```python
from build123d import *

# Parameters (mm, degrees)
SKETCH1_W               = 100
SKETCH1_H               = 100
BOSS_EXTRUDE1_DEPTH     = 50
SHELL1_T                = -10
CUT_EXTRUDE1_DEPTH      = 151
CUT_EXTRUDE1_DEPTH_BACK = 10
SKETCH2_W               = 50
SKETCH2_H               = 15
SKETCH3_W               = 25
SKETCH3_H               = 65
CUT_EXTRUDE2_DEPTH      = 10
SKETCH4_W               = 12.5
SKETCH4_H               = 32.5
CUT_EXTRUDE3_DEPTH      = 10
CUT_EXTRUDE4_START      = -40
SKETCH5_W               = 90
SKETCH5_H               = 90
CUT_EXTRUDE4_DEPTH      = 40
SKETCH6_W               = 6
SKETCH6_H               = 3
BOSS_EXTRUDE2_DEPTH     = 3


with BuildPart() as part:
    # Sketch1 → Boss-Extrude1 (new body)
    with BuildSketch(Plane.XY):
        with Locations((50, 50)):
            Rectangle(SKETCH1_W, SKETCH1_H)
    extrude(amount=BOSS_EXTRUDE1_DEPTH)

    # Shell1
    shell1_openings = [part.faces().sort_by_distance(p)[0] for p in [
        (50, 50, 50),
    ]]
    offset(amount=SHELL1_T, openings=shell1_openings, kind=Kind.INTERSECTION)

    # Sketch2 → Cut-Extrude1 (cut, two sides: drawn at the far end of the back side and taken through both)
    with BuildSketch(Plane.XZ.offset(-CUT_EXTRUDE1_DEPTH_BACK)):
        with Locations((50, 17.5)):
            Rectangle(SKETCH2_W, SKETCH2_H)
    extrude(amount=CUT_EXTRUDE1_DEPTH + CUT_EXTRUDE1_DEPTH_BACK, mode=Mode.SUBTRACT)

    # Sketch3 → Cut-Extrude2 (cut)
    with BuildSketch(Plane.ZY.offset(-100)):
        with Locations((22.5, 59.5)):
            Rectangle(SKETCH3_W, SKETCH3_H)
    extrude(amount=CUT_EXTRUDE2_DEPTH, mode=Mode.SUBTRACT)

    # Sketch4 → Cut-Extrude3 (cut)
    with BuildSketch(Plane(origin=(0, 0, 0), x_dir=(0, 0, -1), z_dir=(1, 0, 0))):
        with Locations((-16.25, 43.25)):
            Rectangle(SKETCH4_W, SKETCH4_H)
    extrude(amount=CUT_EXTRUDE3_DEPTH, mode=Mode.SUBTRACT)

    # Sketch5 → Cut-Extrude4 (cut)
    with BuildSketch(Plane.XY.offset(50).offset(CUT_EXTRUDE4_START)):
        with Locations((50, 50)):
            Rectangle(SKETCH5_W, SKETCH5_H)
    extrude(amount=CUT_EXTRUDE4_DEPTH, mode=Mode.SUBTRACT)

    # Sketch6 → Boss-Extrude2 (add)
    with BuildSketch(Plane.XY.offset(10)):
        with Locations((8, 31.5)):
            Rectangle(SKETCH6_W, SKETCH6_H)
        with Locations((92, 31.5)):
            Rectangle(SKETCH6_W, SKETCH6_H)
    extrude(amount=BOSS_EXTRUDE2_DEPTH)


solid = part.part
```
Build history of the part. All positions in model axes, mm. A direction names the side the tool comes from. Give positions to 0.01 mm unless a question says otherwise; leave off trailing zeros. Loops run counter-clockwise (first coordinate to the right, second up) from the corner with the lowest first, then second, coordinate; pieces in that order, holes last.
Item 1: Which spindle directions (+Z, -Z, +X, -X, +Y, -Y) get a long thin tool onto all of the face, cutting with end or side? Do faces 5 (the face through (2, 27, 16)), 6 (the face through (5, 49, 34)), 7 (the face through (92, 30, 11)), 8 (the face through (5, 31, 11)), 9 (the face through (75, 3, 17)). Say none if no direction does.
Answers follow:
face 5: +X, -X
face 6: +Z
face 7: +Z, +X, -X
face 8: -X
face 9: -Y
Item 2: Flat gauge pins, fed straight in: pin 1 (3.5 mm diameter, centred on y = 31, z = 12, fed in from -X); pin 2 (3 mm diameter, centred on y = 63.5, z = 17.5, fed in from +X); pin 3 (1.5 mm diameter, centred on x = 65.5, z = 17, fed in from -Y). Where does each tip first touch, or does it go through?
Answers follow:
pin 1: stops at x = 5
pin 2: stops at x = 5
pin 3: stops at y = 95
Item 3: Drill centre lines: line 1 (Y direction, x = 74, z = 46.5); line 2 (X direction, y = 84, z = 14). Where is each one in solid material? Low to high.
Answers follow:
line 1: y = 0 to 5, 95 to 100
line 2: x = 0 to 5
Item 4: Slice it at D-D, the plane z = 43.5. List the corners of the cut face in (x, y).
Answers follow:
outline: (0, 0) - (100, 0) - (100, 100) - (0, 100) - close; hole (5, 5) - (95, 5) - (95, 95) - (5, 95) - close
Item 5: Slice it at C-C, the plane y = 65. List the corners of the cut face in (x, z), and give its area (4 significant figures).
Answers follow:
outline: (0, 0) - (100, 0) - (100, 10) - (5, 10) - (5, 50) - (0, 50) - close; (95, 35) - (100, 35) - (100, 50) - (95, 50) - close
area: 1,275 mm2
Item 6: Slice it at B-B, the plane z = 16. List the corners of the cut face in (x, y).
Answers follow:
outline: (0, 0) - (25, 0) - (25, 5) - (5, 5) - (5, 27) - (0, 27) - close; (0, 59.5) - (5, 59.5) - (5, 95) - (95, 95) - (95, 92) - (100, 92) - (100, 100) - (0, 100) - close; (75, 0) - (100, 0) - (100, 27) - (95, 27) - (95, 5) - (75, 5) - close
Item 7: Slice it at A-A, the plane x = 47. List the corners of the cut face in (y, z).
Answers follow:
outline: (0, 0) - (100, 0) - (100, 50) - (95, 50) - (95, 10) - (0, 10) - close; (0, 25) - (5, 25) - (5, 50) - (0, 50) - close
Item 8: Pull direction Y, two halves, no side cores. Call faces 1 (the face through (100, 49, 36)), 2 (the face through (49, 0, 30)), 3 (the face through (98, 27, 22)), 4 (the face through (49, 5, 34)): released by +Y, released by -Y, zero draft, split by the parting line, or undercut.
Answers follow:
face 1: zero draft
face 2: released by -Y
face 3: undercut
face 4: undercut
